The listing builds one solid part. Answer for the finished solid, in the listing's coordinates (mm). A direction names the side the tool comes from. Round coordinates to 2 decimals unless told otherwise and drop trailing zeros. Order: outer loops, then holes, each group sorted by start corner. A loop starts at its lowest first (then second) coordinate and runs counter-clockwise, first axis right, second up. Notation, with made-up numbers: M 44.5,41 L 71.5,41 A10 cw 71.5,58 Z; hole C 79,-31.75 d6. An arc over 180 degrees is marked long. Write item = value, one per line. Start each with the question number.
(1) Each of these flat-tipped pins is pushed along its axis until it touches: pin 1 (6 mm diameter, centred on x = -22, y = -19.5, fed in from +Z); pin 2 (1.6 mm diameter, centred on x = -35, y = -3, fed in from +Z). Where does it stop, or does it pass through?
(2) A straight line is drawn through the part: probe 1 along Z at (x, y) = (-20, -7.75). Find the intervals that lie inside material, in ascending order. Write a range as from..to.
(3) Which of the six approach directions +Z, -Z, +X, -X, +Y, -Y give full straight-line access (tool end or side, diameter ignored) to faces 1 (the face through (-25, -3, 9)), 2 (the face through (-25, -21, 10))?
(4) For a pull along Y with two mould halves and no side action, classify faces 3 (the face through (-25, -13, 10)), 4 (the face through (-25, -30, 5)), 5 (the face through (-25.3, -24, 9.5)), 6 (the face through (-25.3, -4, 9.5)) as released by +Y, released by -Y, zero draft, split by the parting line, or undercut.
(5) A cutting plane is placed at B-B, the plane y = -15. Determine the outline of the cut face in (x, z), and give its area (3 significant figures).
from build123d import *

# Parameters (mm, degrees)
SKETCH1_W           = 50
SKETCH1_H           = 30
BOSS_EXTRUDE1_DEPTH = 10
SKETCH2_W           = 50
SKETCH2_H           = 2
CUT_EXTRUDE3_DEPTH  = 1


with BuildPart() as part:
    # Sketch1 → Boss-Extrude1 (new body)
    with BuildSketch(Plane.XY):
        with Locations((-25, -15)):
            Rectangle(SKETCH1_W, SKETCH1_H)
    extrude(amount=BOSS_EXTRUDE1_DEPTH)

    # Sketch2 → Cut-Extrude3 (cut)
    with BuildSketch(Plane.XY.offset(10)):
        with Locations((-25, -3)):
            Rectangle(SKETCH2_W, SKETCH2_H)
        with Locations((-25, -7)):
            Rectangle(SKETCH2_W, SKETCH2_H)
        with Locations((-25, -11)):
            Rectangle(SKETCH2_W, SKETCH2_H)
        with Locations((-25, -15)):
            Rectangle(SKETCH2_W, SKETCH2_H)
        with Locations((-25, -19)):
            Rectangle(SKETCH2_W, SKETCH2_H)
        with Locations((-25, -23)):
            Rectangle(SKETCH2_W, SKETCH2_H)
        with Locations((-25, -27)):
            Rectangle(SKETCH2_W, SKETCH2_H)
    extrude(amount=-CUT_EXTRUDE3_DEPTH, mode=Mode.SUBTRACT)


solid = part.part
Reported:
q1.pin_1 = 10
q1.pin_2 = 9
q2.probe_1 = 0..9
q3.face_1 = +Z, +X, -X
q3.face_2 = +Z, +X, -X, +Y, -Y
q4.face_3 = zero draft
q4.face_4 = released by -Y
q4.face_5 = undercut
q4.face_6 = undercut
q5.outline = M -50,0 L 0,0 L 0,9 L -50,9 Z
q5.area = 450 mm²
